from build123d import *

# Parameters (mm, degrees)
BOSS_EXTRUDE1_DEPTH = 99.06
SKETCH2_W           = 83.82
SKETCH2_H           = 60.96
CUT_EXTRUDE1_DEPTH  = 86.106
SKETCH3_R           = 1.65
CUT_EXTRUDE2_DEPTH  = 228.6
SKETCH4_R           = 1.7526
CUT_EXTRUDE3_DEPTH  = 228.6


with BuildPart() as part:
    # Sketch1 → Boss-Extrude1 (new body)
    with BuildSketch(Plane(origin=(0, 0, 0), x_dir=(0, 0, -1), z_dir=(1, 0, 0))):
        Polygon((-29.897403577, 26.181538462), (-12.117403577, 26.181538462), (-12.117403577, 21.101538462), (-24.817403577, 21.101538462), (-24.817403577, -39.858461538), (-29.897403577, -39.858461538), align=None)
    extrude(amount=BOSS_EXTRUDE1_DEPTH)

    # Sketch2 → Cut-Extrude1 (cut)
    with BuildSketch(Plane.XY):
        with Locations((49.53, -11.918461538)):
            Rectangle(SKETCH2_W, SKETCH2_H)
    extrude(amount=CUT_EXTRUDE1_DEPTH, mode=Mode.SUBTRACT)

    # Sketch3 → Cut-Extrude2 (cut)
    with BuildSketch(Plane.XY):
        with Locations(Location((96.41, -37.208461538, 0), (0, 0, 180))):
            Circle(SKETCH3_R)
        with Locations(Location((96.41, 17.491538462, 0), (0, 0, 180))):
            Circle(SKETCH3_R)
        with Locations(Location((3.41, 17.491538462, 0), (0, 0, 180))):
            Circle(SKETCH3_R)
        with Locations(Location((3.41, -37.208461538, 0), (0, 0, 180))):
            Circle(SKETCH3_R)
    extrude(amount=CUT_EXTRUDE2_DEPTH, mode=Mode.SUBTRACT)

    # Sketch4 → Cut-Extrude3 (cut)
    with BuildSketch(Plane(origin=(0, 0, 0), x_dir=(1, 0, 0), z_dir=(0, 1, 0))):
        with Locations(Location((7.62, -16.70215043, 0), (0, 0, 90))):
            Circle(SKETCH4_R)
        with Locations(Location((15.24, -16.70215043, 0), (0, 0, 90))):
            Circle(SKETCH4_R)
        with Locations(Location((83.82, -16.70215043, 0), (0, 0, 90))):
            Circle(SKETCH4_R)
        with Locations(Location((91.44, -16.70215043, 0), (0, 0, 90))):
            Circle(SKETCH4_R)
    extrude(amount=CUT_EXTRUDE3_DEPTH, mode=Mode.SUBTRACT)


solid = part.part
Read the model definition and answer for the solid it produces. Units are mm, in the model's axes. A direction names the side the tool comes from. Round coordinates to 2 decimals unless told otherwise and drop trailing zeros. Write each loop counter-clockwise with the first axis right and the second up, starting at its lowest first coordinate (ties: lowest second). Pieces come first, ordered by that corner, then holes. Notation, with made-up numbers: M 7.5,53.5 L 29.5,53.5 A31 ccw 29.5,88.5 Z; hole C 67.25,80.5 d2. An arc over 180 degrees is marked long. Use a Markdown table: item, result.
1) A tool of negligible diameter and unlimited length cuts with its end or side. For faces 5 (the flat face through (4, -39.858, 27)), 6 (the flat face through (49, 21.102, 18)), 7 (the flat face through (91.44, -11, 27)), from which of +Z, -Z, +X, -X, +Y, -Y can it reach the whole face along a straight path? Write none if from no direction.
Answers follow:
| item | result |
|---|---|
| face 5 | +Z, -Z, +X, -X, -Y |
| face 6 | -Z, +X, -X, -Y |
| face 7 | +Z, -Z, -Y |
2) The part is cut by section B-B (x = 15.24). Write down the section's boundary in (y, z), plus the area to 3 significant figures.
Answers follow:
| item | result |
|---|---|
| outline | M 18.56,24.82 L 21.1,24.82 L 21.1,18.45 L 26.18,18.45 L 26.18,29.9 L 18.56,29.9 Z; M 21.1,12.12 L 26.18,12.12 L 26.18,14.95 L 21.1,14.95 Z |
| area | 85.4 mm2 |
3) Flat-ended cylindrical pins translate along their axes: pin 1 (4 mm diameter, centred on x = 29.5, z = 16.5, fed in from -Y); pin 2 (4 mm diameter, centred on x = 63.5, z = 27.5, fed in from -Y). Find the tip coordinate at first contact, or state that the pin passes through.
Answers follow:
| item | result |
|---|---|
| pin 1 | stops at y = 21.1 |
| pin 2 | stops at y = 18.56 |
4) For a pull along Z with two mould halves and no side action, classify faces 1 (the cylindrical face through (2.649, -35.745, 27.322)), 2 (the flat face through (49, 20, 29.897)), 3 (the cylindrical face through (13.5, 23.6, 16.9)), 4 (the flat face through (53, 20, 24.817)) as pulls with the +Z half, pulls with the -Z half, needs draft (parallel to the pull), parting line crosses it, or undercut.
Answers follow:
| item | result |
|---|---|
| face 1 | needs draft |
| face 2 | pulls with the +Z half |
| face 3 | undercut |
| face 4 | pulls with the -Z half |
5) The part is cut by section D-D (z = 16.25). Write down the section's boundary in (x, y), plus the area to 3 significant figures.
Answers follow:
| item | result |
|---|---|
| outline | M 0,21.1 L 5.93,21.1 L 5.93,26.18 L 0,26.18 Z; M 9.31,21.1 L 13.55,21.1 L 13.55,26.18 L 9.31,26.18 Z; M 16.93,21.1 L 82.13,21.1 L 82.13,26.18 L 16.93,26.18 Z; M 85.51,21.1 L 89.75,21.1 L 89.75,26.18 L 85.51,26.18 Z; M 93.13,21.1 L 99.06,21.1 L 99.06,26.18 L 93.13,26.18 Z |
| area | 434 mm2 |
6) Straight lines are drawn through the part: line 1 along Y through (x, z) = (3.41, 28.5); line 2 along X through (y, z) = (-23.5, 28.5); line 3 along Y through (x, z) = (33, 24.25). For each, find the intervals that lie inside material, in ascending order. Write a range as [from, to].
Answers follow:
| item | result |
|---|---|
| line 1 | y = [-39.86, -38.86], [-35.56, 15.84], [19.14, 26.18] |
| line 2 | x = [0, 7.62], [91.44, 99.06] |
| line 3 | y = [21.1, 26.18] |
7) The part is cut by section C-C (x = 3.41). Write down the section's boundary in (y, z), plus the area to 3 significant figures.
Answers follow:
| item | result |
|---|---|
| outline | M -39.86,24.82 L -38.86,24.82 L -38.86,29.9 L -39.86,29.9 Z; M -35.56,24.82 L 15.84,24.82 L 15.84,29.9 L -35.56,29.9 Z; M 19.14,24.82 L 21.1,24.82 L 21.1,12.12 L 26.18,12.12 L 26.18,29.9 L 19.14,29.9 Z |
| area | 366 mm2 |
8) The part is cut by section A-A (y = -3). Write down the section's boundary in (x, z), plus the area to 3 significant figures.
Answers follow:
| item | result |
|---|---|
| outline | M 0,24.82 L 7.62,24.82 L 7.62,29.9 L 0,29.9 Z; M 91.44,24.82 L 99.06,24.82 L 99.06,29.9 L 91.44,29.9 Z |
| area | 77.4 mm2 |
